Here's how the part is built. I have some questions about the finished solid (model axes, mm). Face numbers are marked on the shaded views. A direction names the side the tool comes from. Give positions to 0.01 mm unless a question says otherwise; leave off trailing zeros. Write each loop counter-clockwise with the first axis right and the second up, starting at its lowest first coordinate (ties: lowest second). Pieces come first, ordered by that corner, then holes. Notation, with made-up numbers: (64.5, 29.5) -> (117.5, 29.5) arc R15 cw to (117.5, 48.5) -> close; hole circle Ø11 at (4, -2). An arc over 180 degrees is marked (long way). Return JSON: item names as keys, results as strings.
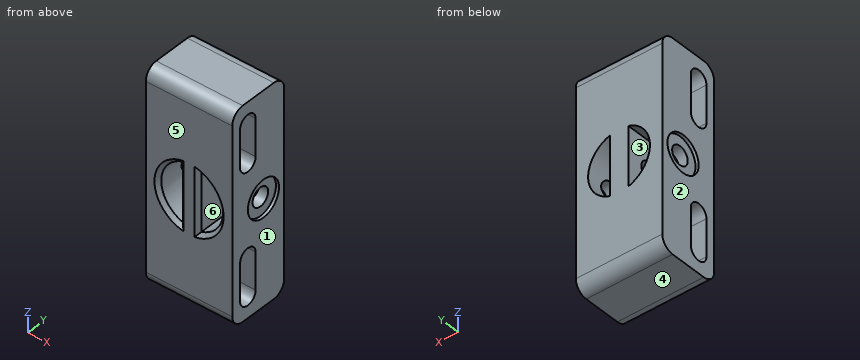
from build123d import *

# Parameters (mm, degrees)
SKETCH_1_W          = 14
SKETCH_1_H          = 34
EXTRUDE_1_DEPTH     = 10
SKETCH_2_R          = 1.5
CUT_EXTRUDE_1_DEPTH = 25.186773245
SKETCH_3_R          = 3
CUT_EXTRUDE_2_DEPTH = 0.5
CUT_EXTRUDE_3_DEPTH = 25.186773286
FILLET_1_R          = 2
CHAMFER_1_SIZE      = 0.6


with BuildPart() as part:
    # 草图1 → 凸台-拉伸1 (new body)
    with BuildSketch(Plane(origin=(0, 0, 0), x_dir=(1, 0, 0), z_dir=(0, 1, 0))):
        Rectangle(SKETCH_1_W, SKETCH_1_H)
        with BuildLine():
            Line((-1.5, 4.769696007), (-1.5, -4.769696007))
            ThreePointArc((-1.5, -4.769696007), (-5, 0), (-1.5, 4.769696007))
        make_face(mode=Mode.SUBTRACT)
        with BuildLine():
            Line((1.5, 4.769696007), (1.5, -4.769696007))
            ThreePointArc((1.5, -4.769696007), (5, 0), (1.5, 4.769696007))
        make_face(mode=Mode.SUBTRACT)
    extrude(amount=EXTRUDE_1_DEPTH)

    # 草图2 → 切除-拉伸1 (cut, through all)
    with BuildSketch(Plane.ZY.offset(7)):
        with Locations((0, 6)):
            Circle(SKETCH_2_R)
    extrude(amount=-CUT_EXTRUDE_1_DEPTH, mode=Mode.SUBTRACT)

    # 草图3 → 切除-拉伸2 (cut)
    with BuildSketch(Plane.ZY.offset(7)):
        with Locations((0, 6)):
            Circle(SKETCH_3_R)
    cut_extrude_2 = extrude(amount=-CUT_EXTRUDE_2_DEPTH, mode=Mode.SUBTRACT)

    # 镜向1: 切除-拉伸2 across plane
    add(cut_extrude_2.mirror(Plane(origin=(0, 0, 0), x_dir=(0, 0, 1), z_dir=(1, 0, 0))), mode=Mode.SUBTRACT)

    # 草图4 → 切除-拉伸3 (cut, through all)
    with BuildSketch(Plane.ZY.offset(7)):
        with BuildLine():
            Line((-13.5, 4.5), (-7.5, 4.5))
            ThreePointArc((-7.5, 4.5), (-6, 3), (-7.5, 1.5))
            Line((-7.5, 1.5), (-13.5, 1.5))
            ThreePointArc((-13.5, 1.5), (-15, 3), (-13.5, 4.5))
        make_face()
        with BuildLine():
            Line((7.5, 1.5), (13.5, 1.5))
            ThreePointArc((13.5, 1.5), (15, 3), (13.5, 4.5))
            Line((13.5, 4.5), (7.5, 4.5))
            ThreePointArc((7.5, 4.5), (6, 3), (7.5, 1.5))
        make_face()
    extrude(amount=-CUT_EXTRUDE_3_DEPTH, mode=Mode.SUBTRACT)

    # 圆角1
    fillet_1_edges = [part.edges().sort_by_distance(p)[0] for p in [
        (0, 10, 17),
        (0, 0, 17),
        (0, 0, -17),
        (0, 10, -17),
    ]]
    fillet(fillet_1_edges, radius=FILLET_1_R)

    # 倒角1
    chamfer_1_edges = [part.edges().sort_by_distance(p)[0] for p in [
        (5, 0, 0),
        (1.5, 0, 0),
        (-5, 0, 0),
        (-1.5, 0, 0),
    ]]
    chamfer(chamfer_1_edges, length=CHAMFER_1_SIZE)


solid = part.part
1. If I drill on line 1 (X direction, y = 3.75, z = -4); line 2 (X direction, y = 2.25, z = 0); line 3 (Y direction, x = 6.65, z = 0), over which ranges is the centre line in solid material (lowest first)? Write a range as [from, to].
Taken from the geometry:
{"line 1": "x = [-7, -3], [-1.5, 1.5], [3, 7]", "line 2": "x = [-7, -5], [-1.5, 1.5], [5, 7]", "line 3": "y = [0, 3], [9, 10]"}
2. Suppose I cut it at D-D, the plane z = 0. Count the separate pieces of the cut face and the enclosed holes in it, and give its area (3 significant figures).
Taken from the geometry:
{"separate pieces": "6", "enclosed holes": "0", "area": "45.3 mm²"}
3. Suppose I cut it at C-C, the plane x = 0.5. List the corners of the cut face in (y, z) for me.
Taken from the geometry:
{"outline": "(0, -15) arc R2 ccw to (2, -17) -> (8, -17) arc R2 ccw to (10, -15) -> (10, 15) arc R2 ccw to (8, 17) -> (2, 17) arc R2 ccw to (0, 15) -> close; hole (1.5, -13.5) arc R1.5 ccw to (4.5, -13.5) -> (4.5, -7.5) arc R1.5 ccw to (1.5, -7.5) -> close; hole (1.5, 7.5) arc R1.5 ccw to (4.5, 7.5) -> (4.5, 13.5) arc R1.5 ccw to (1.5, 13.5) -> close; hole circle Ø3 at (6, 0)"}
4. For pin 1 Ø5 at (y, z) = (6, 0) entering from +X; pin 2 Ø2.5 at (y, z) = (6, 0) entering from +X; pin 3 Ø3.5 at (y, z) = (6, 0) entering from -X, each with a flat end and sliding along its axis, tell me the tip position at first contact or that it passes through.
Taken from the geometry:
{"pin 1": "stops at x = 6.5", "pin 2": "passes through", "pin 3": "stops at x = -6.5"}
5. Which directions (+Z, -Z, +X, -X, +Y, -Y) give clear straight access to the entire face, cutting with the end or side of a thin tool? Please do the marked faces 5 and 6.
Taken from the geometry:
{"face 5": "+Z, -Z, +X, -X, -Y", "face 6": "+Y, -Y"}
6. Suppose I cut it at A-A, the plane z = -11. List the corners of the cut face in (x, y) for me.
Taken from the geometry:
{"outline": "(-7, 0) -> (7, 0) -> (7, 1.5) -> (-7, 1.5) -> close; (-7, 4.5) -> (7, 4.5) -> (7, 10) -> (-7, 10) -> close"}
7. Suppose I cut it at B-B, the plane y = 6. List the corners of the cut face in (x, z) for me.
Taken from the geometry:
{"outline": "(-7, -17) -> (7, -17) -> (7, -3) -> (6.5, -3) -> (6.5, -1.5) -> (4.77, -1.5) arc R5 cw to (1.5, -4.77) -> (1.5, -1.5) -> (-1.5, -1.5) -> (-1.5, -4.77) arc R5 cw to (-4.77, -1.5) -> (-6.5, -1.5) -> (-6.5, -3) -> (-7, -3) -> close; (-7, 3) -> (-6.5, 3) -> (-6.5, 1.5) -> (-4.77, 1.5) arc R5 cw to (-1.5, 4.77) -> (-1.5, 1.5) -> (1.5, 1.5) -> (1.5, 4.77) arc R5 cw to (4.77, 1.5) -> (6.5, 1.5) -> (6.5, 3) -> (7, 3) -> (7, 17) -> (-7, 17) -> close"}
8. If we mould it in two halves opening along X, with no side actions, what happens to the marked faces 1, 2, 3 and 4? For each: released by +X, released by -X, zero draft, split by the parting line, or undercut.
Taken from the geometry:
{"face 1": "released by +X", "face 2": "released by -X", "face 3": "undercut", "face 4": "zero draft"}
